from build123d import *

# Parameters (mm, degrees)
BOSS_EXTRUDE1_DEPTH = 152.4
SKETCH2_R           = 12.7
BOSS_EXTRUDE2_DEPTH = 127
CUT_EXTRUDE1_DEPTH  = 12.7
FILLET1_R           = 6.35


with BuildPart() as part:
    # Sketch1 → Boss-Extrude1 (new body)
    with BuildSketch(Plane.XY):
        with BuildLine():
            Line((-38.1, 0), (-38.1, 50.8))
            Line((-38.1, 50.8), (38.1, 50.8))
            Line((38.1, 50.8), (38.1, 0))
            ThreePointArc((38.1, 0), (0, -38.1), (-38.1, 0))
        make_face()
    extrude(amount=-BOSS_EXTRUDE1_DEPTH)

    # Sketch2 → Boss-Extrude2 (add)
    with BuildSketch(Plane.XY):
        Circle(SKETCH2_R)
    extrude(amount=BOSS_EXTRUDE2_DEPTH)

    # Sketch3 → Cut-Extrude1 (cut)
    with BuildSketch(Plane(origin=(0, 50.8, 0), x_dir=(1, 0, 0), z_dir=(0, 1, 0))):
        with BuildLine():
            Line((5.08, 45.139822986), (5.08, 38.1))
            Line((5.08, 38.1), (-5.08, 38.1))
            Line((-5.08, 38.1), (-5.08, 45.139822986))
            ThreePointArc((-5.08, 45.139822986), (0, 82.55), (5.08, 45.139822986))
        make_face()
    extrude(amount=-CUT_EXTRUDE1_DEPTH, mode=Mode.SUBTRACT)

    # Fillet1
    fillet1_edges = [part.edges().sort_by_distance(p)[0] for p in [
        (0, 50.8, -152.4),
        (-38.1, 25.4, -152.4),
        (0, -38.1, -152.4),
        (-38.1, 25.4, 0),
        (0, 50.8, 0),
        (38.1, 25.4, 0),
        (0, -38.1, 0),
        (38.1, 25.4, -152.4),
        (-38.1, 50.8, -76.2),
        (38.1, 50.8, -76.2),
    ]]
    fillet(fillet1_edges, radius=FILLET1_R)


solid = part.part
Check sheet for the modelled part. Datum: model origin and axes. Units: mm. A direction names the side the tool comes from. Give positions to 0.01 mm unless a question says otherwise; leave off trailing zeros. Loops run counter-clockwise (first coordinate to the right, second up) from the corner with the lowest first, then second, coordinate; pieces in that order, holes last. Notation, with made-up numbers: M -12.75,-10 L 6.25,-10 A22 cw 6.25,0 Z; hole C -36,23.25 d9. An arc over 180 degrees is marked long. Answer as a JSON object with one key per item and string values. Group by question number.
Q1. Cross-section at B-B on z = -63.5. Record the cut outline in (x, y).
Q2. Material ranges on line 1 along X through (y, z) = (44.5, -63.5); line 2 along Z through (x, y) = (1, 44.5); line 3 along Z through (x, y) = (-31, 17), recorded low to high. Write a range as [from, to].
Q3. Cross-section at D-D on z = 41. Record the cut outline in (x, y).
Q4. Release check for a two-part mould opening along X. For faces 3 (the cylindrical face through (0.44, 48.99, -150.49)), 4 (the flat face through (-38.1, 22, -75)), 5 (the flat face through (0, 45, -38.1)) record: released by +X, released by -X, zero draft, split by the parting line, or undercut.
Q5. Cross-section at C-C on y = 28. Record the cut outline in (x, z), then the cut area to 3 significant figures.
Q6. Access from +Z, -Z, +X, -X, +Y, -Y to the whole of each face (thin tool, end or side, straight path). Record for faces 1 (the flat face through (5.08, 45, -42)), 2 (the flat face through (0, 50.8, -91)).
Q7. Cross-section at A-A on x = 0. Record the cut outline in (y, z).
Q8. Go/stop test with flat-tipped pins: P1, Ø4, axis at x = 4.5, y = 25, coming from the +Z side; P2, Ø23, axis at x = 0, z = -63.5, coming from the +Y side; P3, Ø12, axis at x = 27, z = 3, coming from the -Y side; P4, Ø3, axis at x = 1, y = 46, coming from the -Z side. Record where each tip stops, or that it passes through.
Evaluation:
{
 "1": {"outline": "M -38.1,0 A38.1 ccw 38.1,0 L 38.1,44.45 A6.35 ccw 31.75,50.8 L 19.05,50.8 L 19.05,38.1 L -19.05,38.1 L -19.05,50.8 L -31.75,50.8 A6.35 ccw -38.1,44.45 Z"},
 "2": {"line 1": "x = [-38.1, -19.05], [19.05, 38.1]", "line 2": "z = [-152.4, -82.52], [-38.1, 0]", "line 3": "z = [-152.4, 0]"},
 "3": {"outline": "C 0,0 d25.4"},
 "4": {"face 3": "zero draft", "face 4": "released by -X", "face 5": "undercut"},
 "5": {"outline": "M -38.1,-146.05 A6.35 ccw -31.75,-152.4 L 31.75,-152.4 A6.35 ccw 38.1,-146.05 L 38.1,-6.35 A6.35 ccw 31.75,0 L -31.75,0 A6.35 ccw -38.1,-6.35 Z", "area": "11,600 mm2"},
 "6": {"face 1": "+Y", "face 2": "+Z, -Z, +X, -X, +Y"},
 "7": {"outline": "M -38.1,-146.05 A6.35 ccw -31.75,-152.4 L 44.45,-152.4 A6.35 ccw 50.8,-146.05 L 50.8,-82.55 L 38.1,-82.55 L 38.1,-38.1 L 50.8,-38.1 L 50.8,-6.35 A6.35 ccw 44.45,0 L 12.7,0 L 12.7,127 L -12.7,127 L -12.7,0 L -31.75,0 A6.35 ccw -38.1,-6.35 Z"},
 "8": {"P1": "stops at z = 0", "P2": "stops at y = 38.1", "P3": "stops at y = -27.61", "P4": "stops at z = -152.4"}
}
